Source: CAD feature listing. Evaluate the final solid. Frame: model axes, mm. Face numbers are marked on the shaded views. A direction names the side the tool comes from. Give positions to 0.01 mm unless a question says otherwise; leave off trailing zeros. Order: outer loops, then holes, each group sorted by start corner. A loop starts at its lowest first (then second) coordinate and runs counter-clockwise, first axis right, second up. Notation, with made-up numbers: (14.5, -6.5) -> (66.5, -6.5) arc R14 ccw to (66.5, 16.5) -> close; hole circle Ø3 at (22.25, -11.75). An arc over 180 degrees is marked (long way). Answer in a Markdown table with one row per item.
Autodesk Inventor part; units mm, degrees
ref_plane "YZ Plane" through (0, 0, 0) normal (1, 0, 0) x (0, 1, 0)
ref_plane "XZ Plane" through (0, 0, 0) normal (0, 1, 0) x (-1, 0, 0)
ref_plane "XY Plane" through (0, 0, 0) normal (0, 0, 1) x (1, 0, 0)
sketch "Sketch1" plane through (0, 0, 0) normal (0, 1, 0) x (-1, 0, 0)
  line L0 (8.6591, 4.7625) -> (-10.3909, 4.7625)
  line L1 (-10.3909, 4.7625) -> (-10.3909, -4.7625)
  line L2 (-10.3909, -4.7625) -> (8.6591, -4.7625)
  line L3 (8.6591, -4.7625) -> (8.6591, 4.7625)
  circle A0 centre (2.3091, 0) radius 2.3813
  line L4 (-10.3909, 4.7625) -> (-8.8034, 4.7625)
  line L5 (-8.8034, 4.7625) -> (-8.8034, -4.7625)
  line L6 (-8.8034, -4.7625) -> (-10.3909, -4.7625)
  line L7 (-10.3909, -4.7625) -> (-10.3909, 4.7625)
  point P0 (0, 0)
  dimension "d0" = 19.05
  dimension "d1" = 9.525
  dimension "d3" = 4.7625
  dimension "d4" = 12.7
  dimension "d5" = 1.5875
extrude "Extrusion1" add sketch "Sketch1" along normal blind 1.5875 contours L3 L2 L5 L0
extrude "Extrusion2" add sketch "Sketch1" along normal blind 19.05 contours L5 L2 L1 L0
sketch "Sketch2" plane through (10.3909, 0, 4.7625) normal (1, 0, 0) x (0, 0, -1)
  circle A0 centre (4.7625, 12.7) radius 2.3813
  point P0 (4.7625, 0)
  dimension "d10" = 12.7
  dimension "d11" = 4.7625
extrude "Extrusion3" cut sketch "Sketch2" against normal blind 1.5875
properties part number "LBlock"
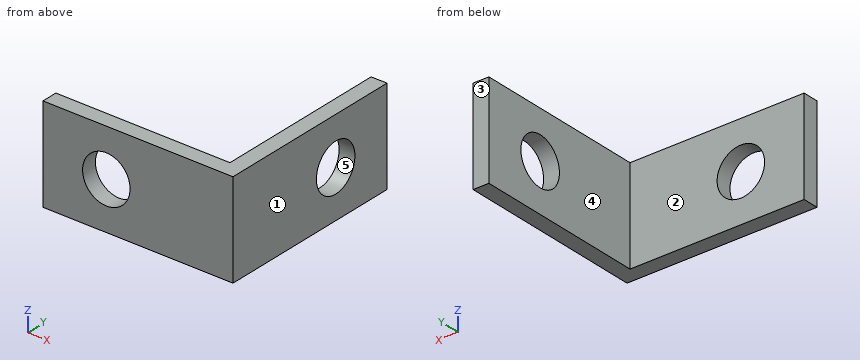
(1) Section query B-B (z = 0). Return the cut outline in (x, y), plus the area to 3 significant figures.
A:
| item | result |
|---|---|
| outline | (-8.66, 0) -> (-4.69, 0) -> (-4.69, 1.59) -> (-8.66, 1.59) -> close; (0.07, 0) -> (10.39, 0) -> (10.39, 10.32) -> (8.8, 10.32) -> (8.8, 1.59) -> (0.07, 1.59) -> close; (8.8, 15.08) -> (10.39, 15.08) -> (10.39, 19.05) -> (8.8, 19.05) -> close |
| area | 42.8 mm^2 |
(2) Section query D-D (y = 6.25). Return the cut outline in (x, z), plus the area to 3 significant figures.
A:
| item | result |
|---|---|
| outline | (8.8, -4.76) -> (10.39, -4.76) -> (10.39, 4.76) -> (8.8, 4.76) -> close |
| area | 15.1 mm^2 |
(3) First-contact query: pin 1 Ø10 at (x, y) = (6, 7.5) entering from -Z; pin 2 Ø3 at (x, z) = (-0.5, -1.5) entering from +Y. Flat tips, straight axial feed; report the tip coordinate or a pass-through.
A:
| item | result |
|---|---|
| pin 1 | stops at z = -4.76 |
| pin 2 | stops at y = 1.59 |
(4) Section query C-C (x = -1). Return the cut outline in (y, z), plus the area to 3 significant figures.
A:
| item | result |
|---|---|
| outline | (0, -4.76) -> (1.59, -4.76) -> (1.59, -1.99) -> (0, -1.99) -> close; (0, 1.99) -> (1.59, 1.99) -> (1.59, 4.76) -> (0, 4.76) -> close |
| area | 8.81 mm^2 |
(5) Pull-direction query (Y, two-part tool) for the marked faces 3, 4 and 5; classes: +Y half, -Y half, draft (parallel to the pull), parting line (faces both ways), or undercut.
A:
| item | result |
|---|---|
| face 3 | +Y half |
| face 4 | draft |
| face 5 | undercut |
(6) Access query for the marked faces 1 and 2. Directions: +Z, -Z, +X, -X, +Y, -Y. A direction counts if a zero-diameter tool reaches every point of the face in a straight line with its end or side. Return the directions, or none.
A:
| item | result |
|---|---|
| face 1 | +Z, -Z, +X, +Y, -Y |
| face 2 | +Z, -Z, -X, +Y |
(7) Ray query, probe 1 along Y at (x, z) = (9.4, 0); probe 2 along X at (y, z) = (9, 0.5); probe 3 along Y at (x, z) = (4, 2.5). Return the intervals inside material, ascending.
A:
| item | result |
|---|---|
| probe 1 | y = 0 to 10.32, 15.08 to 19.05 |
| probe 2 | x = 8.8 to 10.39 |
| probe 3 | y = 0 to 1.59 |
(8) Section query A-A (y = 12.7). Return the cut outline in (x, z), plus the area to 3 significant figures.
A:
| item | result |
|---|---|
| outline | (8.8, -4.76) -> (10.39, -4.76) -> (10.39, -2.38) -> (8.8, -2.38) -> close; (8.8, 2.38) -> (10.39, 2.38) -> (10.39, 4.76) -> (8.8, 4.76) -> close |
| area | 7.56 mm^2 |
